Solid Edge part; units mm, degrees
sketch "Sketch1" plane through (0, 0, 0) normal (0, -1, 0) x (1, 0, 0)
  arc A0 (-110, 35.2168) -> (-64.1736, 56.9886) centre (-105.5765, 85.0207) ccw
  arc A1 (-64.1736, 56.9886) -> (-54.1409, 66.7927) centre (-35.1916, 37.3662) cw
  arc A2 (-54.1409, 66.7927) -> (54.1409, 66.7927) centre (0, -17.2832) cw
  arc A3 (54.1409, 66.7927) -> (64.1736, 56.9886) centre (35.1916, 37.3662) cw
  arc A4 (64.1736, 56.9886) -> (110, 35.2168) centre (105.5765, 85.0207) ccw
  line L0 (110, 35.2168) -> (110, -39.7832)
  arc A5 (110, -39.7832) -> (61.3593, -66.2455) centre (105.5765, -89.5871) ccw
  arc A6 (61.3593, -66.2455) -> (30, -82.6771) centre (31.666, -47.7168) cw
  line L1 (30, -82.6771) -> (-30, -82.6771)
  arc A7 (-61.3593, -66.2455) -> (-30, -82.6771) centre (-31.666, -47.7168) ccw
  arc A8 (-110, -39.7832) -> (-61.3593, -66.2455) centre (-105.5765, -89.5871) cw
  line L2 (-110, 35.2168) -> (-110, -39.7832)
  circle A9 centre (-99.5, 26.2891) radius 2
  circle A10 centre (-99.5, -30.8555) radius 2
  circle A11 centre (99.5, 26.2891) radius 2
  circle A12 centre (99.5, -30.8555) radius 2
extrude "Extrusionsausprägung_2" add sketch "Sketch1" against normal blind 3
properties material "Nylon, allgemein"
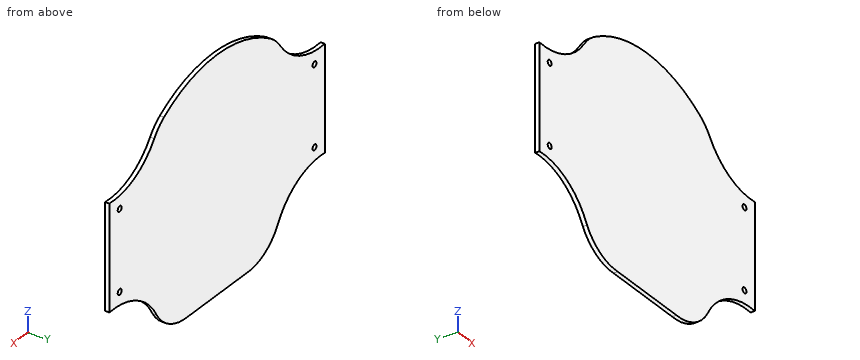
Geometry check sheet. Reference: the model listing, model coordinates, mm. Give positions to 0.01 mm unless a question says otherwise; leave off trailing zeros. Loops run counter-clockwise (first coordinate to the right, second up) from the corner with the lowest first, then second, coordinate; pieces in that order, holes last. Notation, with made-up numbers: (23, 49) -> (31, 49) arc R27 cw to (31, 76) -> close; hole circle Ø10 at (8.25, 13.5). An arc over 180 degrees is marked (long way). Answer in a Markdown table with one row per item. Add a question column.
1) Material ranges on probe 1 along Z at (x, y) = (-99.5, 1.1); probe 2 along Z at (x, y) = (27, 0.4); probe 3 along Z at (x, y) = (-41, 1.25), recorded low to high. Write a range as from..to.
2) Gauge pin test, flat ends, axial feed: P1, Ø1.5, axis at x = 9.5, y = 1, coming from the -Z side; P2, Ø6.5, axis at x = -99.5, z = -30.86, coming from the +Y side; P3, Ø2.5, axis at x = 99.5, z = 26.29, coming from the -Y side. Record the tip position at first contact, or that the pin passes through.
3) Cross-section at B-B on z = 49. Record the boundary of the cut face in (x, y), and give its area (3 significant figures).
4) Cross-section at C-C on x = -90. Record the boundary of the cut face in (y, z), and give its area (3 significant figures).
5) Cross-section at A-A on y = 1.3. Record the boundary of the cut face in (x, z), and give its area (3 significant figures).
Outcome:
| question | item | result |
|---|---|---|
| 1 | probe 1 | z = -39.96..-32.86, -28.86..24.29, 28.29..35.39 |
| 1 | probe 2 | z = -82.68..79 |
| 1 | probe 3 | z = -81.45..73.93 |
| 2 | P1 | stops at z = -82.68 |
| 2 | P2 | stops at y = 3 |
| 2 | P3 | passes through |
| 3 | outline | (-70.9, 0) -> (70.9, 0) -> (70.9, 3) -> (-70.9, 3) -> close |
| 3 | area | 425 mm^2 |
| 4 | outline | (0, -42.08) -> (3, -42.08) -> (3, 37.51) -> (0, 37.51) -> close |
| 4 | area | 239 mm^2 |
| 5 | outline | (-110, -39.78) arc R50 cw to (-61.36, -66.25) arc R35 ccw to (-30, -82.68) -> (30, -82.68) arc R35 ccw to (61.36, -66.25) arc R50 cw to (110, -39.78) -> (110, 35.22) arc R50 cw to (64.17, 56.99) arc R35 ccw to (54.14, 66.79) arc R100 ccw to (-54.14, 66.79) arc R35 ccw to (-64.17, 56.99) arc R50 cw to (-110, 35.22) -> close; hole circle Ø4 at (-99.5, -30.86); hole circle Ø4 at (-99.5, 26.29); hole circle Ø4 at (99.5, -30.86); hole circle Ø4 at (99.5, 26.29) |
| 5 | area | 27,700 mm^2 |
